The drawing under review shows one solid part. Ordinate dimensions are in mm from its lowest x, y, z. Give positions to 0.01 mm unless a question says otherwise; leave off trailing zeros. Order: outer loops, then holes, each group sorted by start corner. A loop starts at its lowest first (then second) coordinate and runs counter-clockwise, first axis right, second up. Notation, with made-up numbers: (11, -32.5) -> (29, -32.5) arc R5 ccw to (29, -26.5) -> close; hole circle Ø8 at (23.5, 46.5). An arc over 180 degrees is marked (long way). One line per item, written item: value.
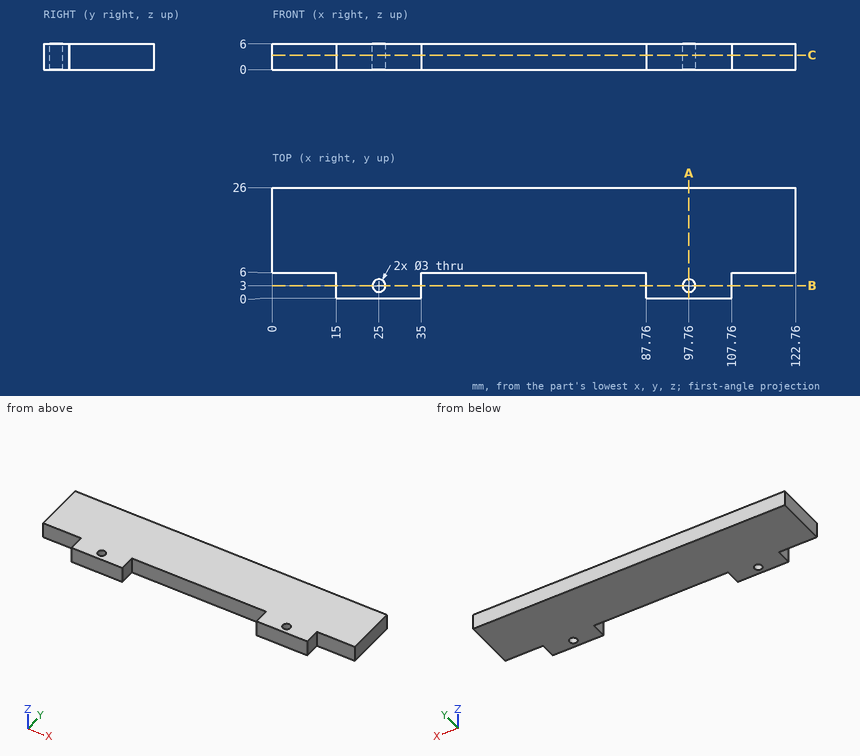
Item 1: Add section C-C on z = 3.4. Give the boundary of the cut face in (x, y), plus the area to 3 significant figures.
Returned:
outline: (0, 6) -> (15, 6) -> (15, 0) -> (35, 0) -> (35, 6) -> (87.76, 6) -> (87.76, 0) -> (107.76, 0) -> (107.76, 6) -> (122.76, 6) -> (122.76, 26) -> (0, 26) -> close; hole circle Ø3 at (25, 3); hole circle Ø3 at (97.76, 3)
area: 2,680 mm²
Item 2: Clearance check with flat-ended pins moving along their axes: P1, Ø1.8, axis at y = 3.5, z = 2, coming from the +X side; P2, Ø1.8, axis at x = 10.5, z = 4.5, coming from the -Y side; P3, Ø1.8, axis at y = 3, z = 1.5, coming from the -X side; P4, Ø2.5, axis at x = 25, y = 3, coming from the -Z side. State where each tip first meets the part, or that it passes through.
Returned:
P1: x = 107.76
P2: y = 6
P3: x = 15
P4: through
Item 3: Add section B-B on y = 3. Give the boundary of the cut face in (x, z).
Returned:
outline: (15, 0) -> (23.5, 0) -> (23.5, 6) -> (15, 6) -> close; (26.5, 0) -> (35, 0) -> (35, 6) -> (26.5, 6) -> close; (87.76, 0) -> (96.26, 0) -> (96.26, 6) -> (87.76, 6) -> close; (99.26, 0) -> (107.76, 0) -> (107.76, 6) -> (99.26, 6) -> close
Item 4: To check wall thickness, follow line 1 along Y through (x, z) = (97.76, 1.85); line 2 along X through (y, z) = (4.75, 0.85); line 3 along X through (y, z) = (1.75, 2.85). State the ranges of each line that lie inside material, in increasing order. Write a range as from..to.
Returned:
line 1: 0..1.5, 4.5..26
line 2: 15..35, 87.76..107.76
line 3: 15..24.17, 25.83..35, 87.76..96.93, 98.59..107.76
Item 5: Add section A-A on x = 97.76. Give the boundary of the cut face in (y, z).
Returned:
outline: (0, 0) -> (1.5, 0) -> (1.5, 6) -> (0, 6) -> close; (4.5, 0) -> (26, 0) -> (26, 6) -> (4.5, 6) -> close
